For this review, take the finished solid that the model builds, in its own axes (mm). A direction names the side the tool comes from. Round coordinates to 2 decimals unless told otherwise and drop trailing zeros. Loops run counter-clockwise (first coordinate to the right, second up) from the corner with the lowest first, then second, coordinate; pieces in that order, holes last.
1) Take a section at A-A (y = 40). State the section outline as (x, z) points, then the cut area to 3 significant figures.
2) Tool access review of faces 4 (the flat face through (-103, 22, 1.524)), 5 (the flat face through (-103, 26.662, 12)), 6 (the flat face through (-96.214, 35, 12)): name each direction out of +Z, -Z, +X, -X, +Y, -Y from which nothing blocks a thin tool from reaching the whole face with its end or side.
3) Take a section at D-D (y = 18.5). State the section outline as (x, z) points.
4) Take a section at C-C (z = 8.25). State the section outline as (x, y) points, then the cut area to 3 significant figures.
5) Mouldability with a two-part tool opening along Y and no side actions: class faces 1 (the cylindrical face through (-101.863, 28.661, 11.521)), 2 (the flat face through (-103, 43.122, 6)), 3 (the flat face through (-101, 42, 0)) as pulls with the +Y half, pulls with the -Y half, needs draft (parallel to the pull), parting line crosses it, or undercut.
6) Insertion check: pin 1 (0.8 mm diameter, centred on y = 19, z = 0.5, fed in from +X); pin 2 (1.5 mm diameter, centred on y = 42.5, z = 1.5, fed in from +X); pin 3 (0.5 mm diameter, centred on x = -100.5, z = 11.5, fed in from -Y). Each pin has a flat end and moves straight along its axis. Give the tip position at first contact, or say it passes through.
7) Wall thickness on L1, parallel to Z at x = -105, y = 42.5; L2, parallel to Z at x = -109.5, y = 7; L3, parallel to X at y = 37, z = 1.25: over which ranges is each line inside the solid? List them lowest first.
8) Take a section at B-B (x = -100.5). State the section outline as (y, z) points.
```python
from build123d import *

# Parameters (mm, degrees)
BOSS_EXTRUDE3_DEPTH = 12.2936
CUT_EXTRUDE3_DEPTH  = 14.3002
SKETCH3_R           = 1.8923
SKETCH3_R_2         = 4.16814
CUT_EXTRUDE4_DEPTH  = 14.3002


with BuildPart() as part:
    # Sketch1 → Boss-Extrude3 (new body)
    with BuildSketch(Plane.XY):
        Polygon((-110.51464309, 1.262410177), (-96.21444309, 1.262410177), (-96.21444309, 43.121610177), (-85.230380887, 60.035582724), (-85.230380887, 62.924026373), (-94.120096356, 62.924026373), (-94.749967174, 82.424781559), (-97.744268584, 82.424781559), (-110.51464309, 43.121610177), align=None)
    extrude(amount=BOSS_EXTRUDE3_DEPTH)

    # Sketch2 → Cut-Extrude3 (cut)
    with BuildSketch(Plane(origin=(-96.21444309, 0, 0), x_dir=(0, 0, -1), z_dir=(1, 0, 0))):
        Polygon((-12.2936, 26.662410177), (-12.2936, 1.262410177), (-10.7696, 1.262410177), (-1.524, 1.262410177), (-1.524, 43.121610177), (-10.7696, 43.121610177), (-10.7696, 26.662410177), align=None)
    extrude(amount=-CUT_EXTRUDE3_DEPTH, mode=Mode.SUBTRACT)

    # Sketch3 → Cut-Extrude4 (cut)
    with BuildSketch(Plane(origin=(0, 0, 0), x_dir=(-1, 0, 0), z_dir=(0, 0, -1))):
        with Locations((103.36454309, 5.529610177)):
            Circle(SKETCH3_R)
        with Locations((103.36454309, 29.812010177)):
            Circle(SKETCH3_R)
        with Locations((103.36454309, 17.035810177)):
            Circle(SKETCH3_R_2)
    extrude(amount=-CUT_EXTRUDE4_DEPTH, mode=Mode.SUBTRACT)


solid = part.part
```
Response:
1. outline: (-110.51, 0) - (-96.21, 0) - (-96.21, 1.52) - (-110.51, 1.52) - close; (-110.51, 10.77) - (-96.21, 10.77) - (-96.21, 12.29) - (-110.51, 12.29) - close
1. area: 43.6 mm2
2. face 4: +X, -X, -Y
2. face 5: +Z, +X, -X, -Y
2. face 6: +Z, -Z, +X, -Y
3. outline: (-110.51, 0) - (-107.27, 0) - (-107.27, 1.52) - (-110.51, 1.52) - close; (-99.46, 0) - (-96.21, 0) - (-96.21, 1.52) - (-99.46, 1.52) - close
4. outline: (-110.51, 43.12) - (-96.21, 43.12) - (-85.23, 60.04) - (-85.23, 62.92) - (-94.12, 62.92) - (-94.75, 82.42) - (-97.74, 82.42) - close
4. area: 470 mm2
5. face 1: undercut
5. face 2: pulls with the -Y half
5. face 3: needs draft
6. pin 1: stops at x = -96.21
6. pin 2: stops at x = -96.13
6. pin 3: stops at y = 26.66
7. L1: z = 0 to 1.52, 10.77 to 12.29
7. L2: z = 0 to 1.52
7. L3: x = -110.51 to -96.21
8. outline: (1.26, 0) - (14.01, 0) - (14.01, 1.52) - (1.26, 1.52) - close; (20.06, 0) - (73.94, 0) - (73.94, 12.29) - (26.66, 12.29) - (26.66, 10.77) - (43.12, 10.77) - (43.12, 1.52) - (20.06, 1.52) - close
